Could you check a few things on this drawing? It's one solid part, dimensions in mm from its lowest x, y, z. A direction names the side the tool comes from. Give positions to 0.01 mm unless a question says otherwise; leave off trailing zeros. Loops run counter-clockwise (first coordinate to the right, second up) from the corner with the lowest first, then second, coordinate; pieces in that order, holes last.
1. Imagine slicing it at C-C (x = 3.5). List the corners of the cut face in (y, z) for me, plus the area to 3 significant figures.
2. For the marked faces 1, 2 and 3, which set-ups out of +Z, -Z, +X, -X, +Y, -Y let a thin tool reach every point of the face, with its end or its side?
3. For P1, Ø1.5, axis at y = 5, z = 4, coming from the -X side; P2, Ø3, axis at y = 12.5, z = 6, coming from the -X side; P3, Ø1, axis at x = 7, z = 4, coming from the -Y side, each with a flat end and sliding along its axis, tell me the tip position at first contact or that it passes through.
4. I need wall thicknesses on line 1 along X through (y, z) = (18.75, 6); line 2 along Z through (x, y) = (12.75, 9); line 3 along Y through (x, z) = (16.5, 7). Which ranges of each line are inside material? Lowest first, please.
5. Imagine slicing it at A-A (z = 6). List the corners of the cut face in (x, y) for me.
6. Imagine slicing it at D-D (y = 9). List the corners of the cut face in (x, z) for me.
7. Thinking about a two-plate mould opening in X: for the marked faces 4, 5, 6 and 7, which applies, +X half, -X half, draft (parallel to the pull), parting line (faces both ways), or undercut?
8. Imagine slicing it at B-B (y = 25.5). List the corners of the cut face in (x, z) for me, plus the area to 3 significant figures.
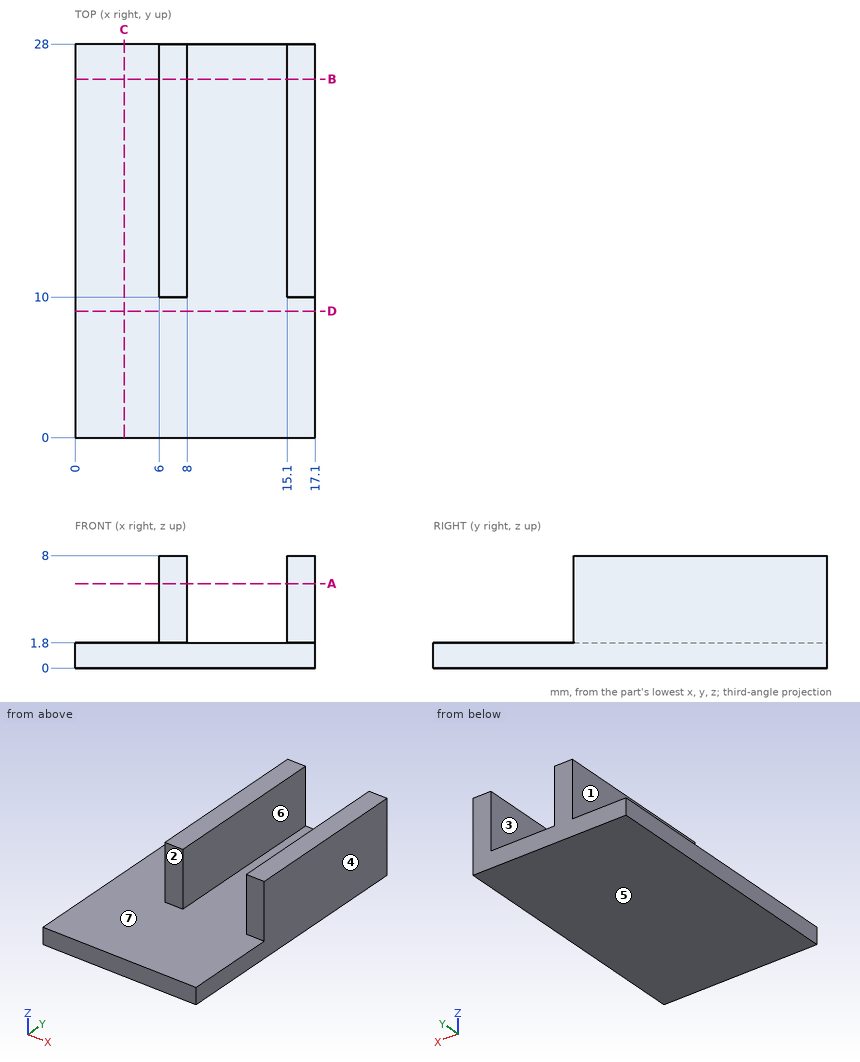
Derived:
1. outline: (0, 0) - (28, 0) - (28, 1.8) - (0, 1.8) - close
1. area: 50.4 mm2
2. face 1: +Z, -X, +Y, -Y
2. face 2: +Z, +X, -X, -Y
2. face 3: +Z, +Y, -Y
3. P1: passes through
3. P2: stops at x = 6
3. P3: stops at y = 10
4. line 1: x = 6 to 8, 15.1 to 17.1
4. line 2: z = 0 to 1.8
4. line 3: y = 10 to 28
5. outline: (6, 10) - (8, 10) - (8, 28) - (6, 28) - close; (15.1, 10) - (17.1, 10) - (17.1, 28) - (15.1, 28) - close
6. outline: (0, 0) - (17.1, 0) - (17.1, 1.8) - (0, 1.8) - close
7. face 4: +X half
7. face 5: draft
7. face 6: undercut
7. face 7: undercut
8. outline: (0, 0) - (17.1, 0) - (17.1, 8) - (15.1, 8) - (15.1, 1.8) - (8, 1.8) - (8, 8) - (6, 8) - (6, 1.8) - (0, 1.8) - close
8. area: 55.6 mm2
